Design review of the part built by this model. Coordinates are the model's own, in mm. A direction names the side the tool comes from. Coordinates: 2 decimals unless noted, no trailing zeros. Write each loop counter-clockwise with the first axis right and the second up, starting at its lowest first coordinate (ties: lowest second). Pieces come first, ordered by that corner, then holes. Notation, with made-up numbers: M 16.25,65 L 70.25,65 A19 ccw 70.25,72 Z; hole C 64.5,51 d1. An arc over 180 degrees is marked long. Return JSON: item names as keys, results as strings. Group by question number.
```python
from build123d import *

# Parameters (mm, degrees)
BOSS_EXTRUDE1_DEPTH = 12
SKETCH2_R           = 8.948929172
BOSS_EXTRUDE2_DEPTH = 3
SKETCH3_R           = 3.175
CUT_EXTRUDE1_DEPTH  = 23
SKETCH4_R           = 6
CUT_EXTRUDE2_DEPTH  = 13


with BuildPart() as part:
    # Sketch1 → Boss-Extrude1 (new body)
    with BuildSketch(Plane(origin=(0, 0, 0), x_dir=(0, 0, -1), z_dir=(1, 0, 0))):
        Polygon((8.948929172, 0), (4.474464586, 7.75), (-4.474464586, 7.75), (-8.948929172, 0), (-4.474464586, -7.75), (4.474464586, -7.75), align=None)
    extrude(amount=BOSS_EXTRUDE1_DEPTH)

    # Sketch2 → Boss-Extrude2 (add)
    with BuildSketch(Plane(origin=(12, 0, 0), x_dir=(0, 0, -1), z_dir=(1, 0, 0))):
        Circle(SKETCH2_R)
    extrude(amount=BOSS_EXTRUDE2_DEPTH)

    # Sketch3 → Cut-Extrude1 (cut)
    with BuildSketch(Plane(origin=(15, 0, 0), x_dir=(0, 0, -1), z_dir=(1, 0, 0))):
        Circle(SKETCH3_R)
    extrude(amount=-CUT_EXTRUDE1_DEPTH, mode=Mode.SUBTRACT)

    # Sketch4 → Cut-Extrude2 (cut)
    with BuildSketch(Plane(origin=(15, 0, 0), x_dir=(0, 0, -1), z_dir=(1, 0, 0))):
        Circle(SKETCH4_R)
    extrude(amount=-CUT_EXTRUDE2_DEPTH, mode=Mode.SUBTRACT)


solid = part.part
```
Item 1: Machinability: for faces 5 (the flat face through (12, 4, 7)), 6 (the flat face through (12, -8, 0)), 7 (the flat face through (5.92, -3.93, -6.68)), 8 (the cylindrical face through (9, 0, 6)), which of the approach directions +Z, -Z, +X, -X, +Y, -Y give a long, thin tool a straight path to every point of the face, cutting with its end or side? Answer none if there is none.
Item 2: Add section C-C (y = 1.25). Write out the cut boundary in (x, z).
Item 3: Add section D-D (x = 8.75). Write out the cut boundary in (y, z).
Item 4: Add section B-B (z = 0). Write out the cut boundary in (x, y) (3 decimals).
Item 5: The part is to be moulded in two halves that separate along Y. For faces 1 (the flat face through (5.916, 3.821, -6.743)), 2 (the cylindrical face through (1.01, -3.1, 0.69)), 3 (the flat face through (12, -4, -7)), 4 (the flat face through (5.916, -3.821, 6.743)), say which applies: pulls with the +Y half, pulls with the -Y half, needs draft (parallel to the pull), parting line crosses it, or undercut.
Item 6: Add section A-A (x = 1.5). Write out the cut boundary in (y, z) (3 decimals).
Item 7: For line 1 (Y direction, x = 10.25, z = 0); line 2 (X direction, y = -2, z = 4.75); line 3 (Z direction, x = 9, y = -4.25), list the stretches that pass through material, from the lowest coordinate up.
Item 8: For pin 1 (1.3 mm diameter, centred on y = -3, z = 6.5, fed in from -X); pin 2 (8 mm diameter, centred on x = 13.5, y = 5.5, fed in from -Z); pin 3 (4 mm diameter, centred on x = 3, z = 2.5, fed in from +Y); pin 4 (1 mm diameter, centred on y = 8.5, z = -1.5, fed in from -X), all flat-tipped, find the tip position at first contact; note any pin that passes through.
Geometry check:
{
 "1": {"face 5": "+Z, -X, +Y", "face 6": "+Z, -Z, -X, -Y", "face 7": "-Z, -X, -Y", "face 8": "+X"},
 "2": {"outline": "M 0,-8.23 L 12,-8.23 L 12,-8.86 L 15,-8.86 L 15,-5.87 L 2,-5.87 L 2,-2.92 L 0,-2.92 Z; M 0,2.92 L 2,2.92 L 2,5.87 L 15,5.87 L 15,8.86 L 12,8.86 L 12,8.23 L 0,8.23 Z"},
 "3": {"outline": "M -7.75,-4.47 L 0,-8.95 L 7.75,-4.47 L 7.75,4.47 L 0,8.95 L -7.75,4.47 Z; hole C 0,0 d12"},
 "4": {"outline": "M 0,-7.75 L 12,-7.75 L 12,-8.949 L 15,-8.949 L 15,-6 L 2,-6 L 2,-3.175 L 0,-3.175 Z; M 0,3.175 L 2,3.175 L 2,6 L 15,6 L 15,8.949 L 12,8.949 L 12,7.75 L 0,7.75 Z"},
 "5": {"face 1": "pulls with the +Y half", "face 2": "undercut", "face 3": "needs draft", "face 4": "pulls with the -Y half"},
 "6": {"outline": "M -7.75,-4.474 L 0,-8.949 L 7.75,-4.474 L 7.75,4.474 L 0,8.949 L -7.75,4.474 Z; hole C 0,0 d6.35"},
 "7": {"line 1": "-7.75 to -6, 6 to 7.75", "line 2": "0 to 2", "line 3": "-6.5 to -4.24, 4.24 to 6.5"},
 "8": {"pin 1": "x = 0", "pin 2": "z = -8.82", "pin 3": "y = 7.75", "pin 4": "x = 12"}
}
